CAD build for the part. Positions are in the model's coordinates, mm. Face numbers are marked on the shaded views. A direction names the side the tool comes from. Give positions to 0.01 mm unless a question says otherwise; leave off trailing zeros. Loops run counter-clockwise (first coordinate to the right, second up) from the corner with the lowest first, then second, coordinate; pieces in that order, holes last. Notation, with made-up numbers: (-24, 0) - (34, 0) arc R19 ccw to (34, 9) - close; hole circle Ø4 at (-36.5, 79). An arc over 180 degrees is marked (long way). Return JSON: item names as keys, results as strings.
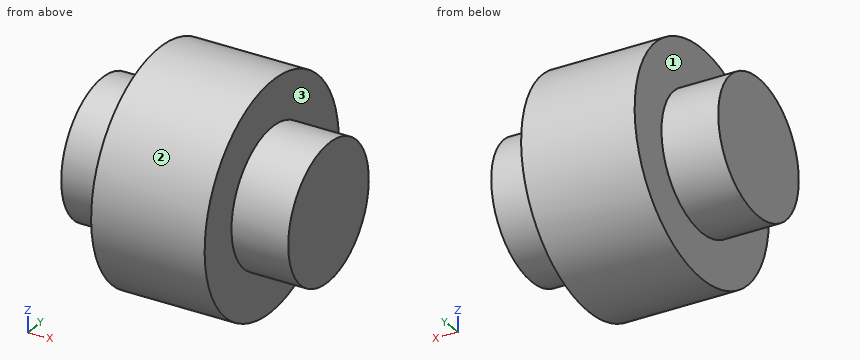
from build123d import *

# Parameters (mm, degrees)
SKETCH1_R           = 7.62
BOSS_EXTRUDE1_DEPTH = 25.4
SKETCH2_R           = 12.7
BOSS_EXTRUDE2_DEPTH = 6.35


with BuildPart() as part:
    # Sketch1 → Boss-Extrude1 (new body)
    with BuildSketch(Plane(origin=(0, 0, 0), x_dir=(0, 0, -1), z_dir=(1, 0, 0))):
        Circle(SKETCH1_R)
    extrude(amount=-BOSS_EXTRUDE1_DEPTH)

    # Sketch2 → Boss-Extrude2 (add, symmetric)
    with BuildSketch(Plane(origin=(-12.7, 0, 0), x_dir=(0, 0, -1), z_dir=(1, 0, 0))):
        Circle(SKETCH2_R)
    extrude(amount=BOSS_EXTRUDE2_DEPTH, both=True)


solid = part.part
1. Cut at A-A, the plane z = 0. Write the cut outline in (x, y), plus the area to 3 significant figures.
Values follow:
{"outline": "(-25.4, -7.62) - (-19.05, -7.62) - (-19.05, -12.7) - (-6.35, -12.7) - (-6.35, -7.62) - (0, -7.62) - (0, 7.62) - (-6.35, 7.62) - (-6.35, 12.7) - (-19.05, 12.7) - (-19.05, 7.62) - (-25.4, 7.62) - close", "area": "516 mm²"}
2. Cut at D-D, the plane z = 8.75. Write the cut outline in (x, y).
Values follow:
{"outline": "(-19.05, -9.2) - (-6.35, -9.2) - (-6.35, 9.2) - (-19.05, 9.2) - close"}
3. Drill centre lines: probe 1 along X at (y, z) = (11.5, 1); probe 2 along Z at (x, y) = (-12, 0.25); probe 3 along Z at (x, y) = (-20.75, -4.75). Where is each one in solid material? Low to high.
Values follow:
{"probe 1": "x = -19.05 to -6.35", "probe 2": "z = -12.7 to 12.7", "probe 3": "z = -5.96 to 5.96"}
4. Cut at C-C, the plane x = -13.5. Write the cut outline in (y, z).
Values follow:
{"outline": "circle Ø25.4 at (0, 0)"}
5. Drop flat-ended pins along their axis: P1, Ø2, axis at x = -19, y = 2.5, coming from the -Z side; P2, Ø10, axis at y = 8.5, z = -8.5, coming from the +X side; P3, Ø12, axis at x = -17.5, z = 9.5, coming from the +Y side; P4, Ø10, axis at x = -16, y = 8.5, coming from the +Z side. Give the stop position or say it passes through.
Values follow:
{"P1": "stops at z = -12.61", "P2": "stops at x = 0", "P3": "stops at y = 12.21", "P4": "stops at z = 12.21"}
6. Which spindle directions (+Z, -Z, +X, -X, +Y, -Y) get a long thin tool onto all of the face, cutting with end or side? Do the marked faces 1, 2 and 3. Say none if no direction does.
Values follow:
{"face 1": "-X", "face 2": "+X, -X", "face 3": "+X"}
